```python
from build123d import *

# Parameters (mm, degrees)
SKETCH1_R           = 6.25
BOSS_EXTRUDE1_DEPTH = 5
BOSS_EXTRUDE2_DEPTH = 2.5


with BuildPart() as part:
    # Sketch1 → Boss-Extrude1 (new body, symmetric)
    with BuildSketch(Plane.XY):
        with BuildLine():
            ThreePointArc((14.68337521, -5), (23.5795956, -2.206380053), (19, 5.916079783))
            Line((19, 5.916079783), (1.5, 8.874119675))
            ThreePointArc((1.5, 8.874119675), (0.214418855, 8.997445446), (-1.075577539, 8.935498473))
            ThreePointArc((-1.075577539, 8.935498473), (-12.706895621, 6.277711403), (-23.530140222, 1.256877932))
            Line((-23.530140222, 1.256877932), (-24.557036845, 2.973118977))
            Line((-24.557036845, 2.973118977), (-34.854483116, -3.188260762))
            Line((-34.854483116, -3.188260762), (-29.72, -11.769465988))
            ThreePointArc((-29.72, -11.769465988), (-18.962777108, -7.283193101), (-7.556000741, -4.889463447))
            ThreePointArc((-7.556000741, -4.889463447), (-1.513896416, -8.871759557), (5.50692712, -7.118549971))
            Line((5.50692712, -7.118549971), (14.68337521, -5))
        make_face()
        Circle(SKETCH1_R, mode=Mode.SUBTRACT)
    extrude(amount=BOSS_EXTRUDE1_DEPTH, both=True)

    # Sketch2 → Boss-Extrude2 (add, symmetric)
    with BuildSketch(Plane.XY):
        with BuildLine():
            ThreePointArc((-22.221689741, -8.394920516), (-24.639151754, -9.353488219), (-27.014289175, -10.412590129))
            Line((-27.014289175, -10.412590129), (-24.649285993, -15.128581404))
            ThreePointArc((-24.649285993, -15.128581404), (-21.175329825, -16.33341689), (-19.970494339, -12.859460723))
            Line((-19.970494339, -12.859460723), (-22.221689741, -8.394920516))
        make_face()
    extrude(amount=BOSS_EXTRUDE2_DEPTH, both=True)


solid = part.part
```
Build history of the part. All positions in model axes, mm. A direction names the side the tool comes from. Round coordinates to 2 decimals unless told otherwise and drop trailing zeros. Order: outer loops, then holes, each group sorted by start corner. A loop starts at its lowest first (then second) coordinate and runs counter-clockwise, first axis right, second up. Notation, with made-up numbers: (76.5, 53.25) - (109.5, 53.25) arc R28 cw to (109.5, 86.25) - close; hole circle Ø6 at (7, 88). An arc over 180 degrees is marked (long way). Use a Markdown table: item, result.
1) Tool access for faces 1 (the face through (-24.036, 2.103, 0.07)), 2 (the face through (-25.848, -12.738, 0.035)), 3 (the face through (-6, -4, -5)): list every direction of +Z, -Z, +X, -X, +Y, -Y with a clear straight run to the whole face (end or side of a thin tool).
Recorded:
| item | result |
|---|---|
| face 1 | +Z, -Z, +Y |
| face 2 | +Z, -Z, -Y |
| face 3 | -Z, +X, -X, +Y, -Y |
2) Saw through at D-D on z = -3.5. Write the cut outline in (x, y).
Recorded:
| item | result |
|---|---|
| outline | (-34.85, -3.19) - (-29.72, -11.77) arc R62 cw to (-7.56, -4.89) arc R9 ccw to (5.51, -7.12) - (14.68, -5) arc R6 ccw (long way) to (19, 5.92) - (1.5, 8.87) arc R9 ccw to (-1.08, 8.94) arc R57 ccw to (-23.53, 1.26) - (-24.56, 2.97) - close; hole circle Ø12.5 at (0, 0) |
3) Saw through at B-B on y = -0.75. Write the cut outline in (x, z), and give its area (3 significant figures).
Recorded:
| item | result |
|---|---|
| outline | (-30.78, -5) - (-6.2, -5) - (-6.2, 5) - (-30.78, 5) - close; (6.2, -5) - (23.95, -5) - (23.95, 5) - (6.2, 5) - close |
| area | 423 mm² |
4) Flat gauge pins, fed straight in: pin 1 Ø2 at (x, y) = (-23.5, -14) entering from -Z; pin 2 Ø2 at (x, y) = (-23, -13) entering from +Z; pin 3 Ø3 at (y, z) = (-3, 2.5) entering from +X; pin 4 Ø4 at (x, y) = (-6.5, -11) entering from +Z. Where does each tip first touch, or does it go through?
Recorded:
| item | result |
|---|---|
| pin 1 | stops at z = -2.5 |
| pin 2 | stops at z = 2.5 |
| pin 3 | stops at x = 23.81 |
| pin 4 | passes through |
5) Wall check: L1, parallel to Y at x = 0, z = 1; L2, parallel to X at y = -11, z = 0.5; L3, parallel to Y at x = -20.5, z = 0.75. Give the ranges that are in metal, low to high.
Recorded:
| item | result |
|---|---|
| L1 | y = -9 to -6.25, 6.25 to 9 |
| L2 | x = -30.18 to -28.23, -26.72 to -20.91 |
| L3 | y = -15.86 to -11.81, -7.78 to 2.95 |
6) Saw through at A-A on x = 0. Write the cut outline in (y, z), and give its area (3 significant figures).
Recorded:
| item | result |
|---|---|
| outline | (-9, -5) - (-6.25, -5) - (-6.25, 5) - (-9, 5) - close; (6.25, -5) - (9, -5) - (9, 5) - (6.25, 5) - close |
| area | 55.0 mm² |
7) Saw through at C-C on z = 0. Write the cut outline in (x, y), and give its area (3 significant figures).
Recorded:
| item | result |
|---|---|
| outline | (-34.85, -3.19) - (-29.72, -11.77) arc R62 cw to (-27.01, -10.41) - (-24.65, -15.13) arc R2.6 ccw to (-19.97, -12.86) - (-22.22, -8.39) arc R62 cw to (-7.56, -4.89) arc R9 ccw to (5.51, -7.12) - (14.68, -5) arc R6 ccw (long way) to (19, 5.92) - (1.5, 8.87) arc R9 ccw to (-1.08, 8.94) arc R57 ccw to (-23.53, 1.26) - (-24.56, 2.97) - close; hole circle Ø12.5 at (0, 0) |
| area | 639 mm² |
8) Pull direction Y, two halves, no side cores. Call faces 4 (the face through (10.031, -6.074, 0.07)), 5 (the face through (23.523, -2.345, 0.07)), 6 (the face through (-23, -12, -2.5)), 7 (the face through (-21.08, -10.66, 0.04)): pulls with the +Y half, pulls with the -Y half, needs draft (parallel to the pull), parting line crosses it, or undercut.
Recorded:
| item | result |
|---|---|
| face 4 | pulls with the -Y half |
| face 5 | parting line crosses it |
| face 6 | needs draft |
| face 7 | undercut |
